Part model, mm, in its own coordinate system. A direction names the side the tool comes from. Round coordinates to 2 decimals unless told otherwise and drop trailing zeros. Loops run counter-clockwise (first coordinate to the right, second up) from the corner with the lowest first, then second, coordinate; pieces in that order, holes last.
1) Mould opens along Z. For faces 1 (the flat face through (-1.052, 23.271, 3.355)), 2 (the cylindrical face through (0.69, 9.39, 3.1)), 3 (the flat face through (-3.43, 23.27, 0.77)), 4 (the flat face through (0, 0, 0)) say: +Z half, -Z half, draft (parallel to the pull), parting line (faces both ways), or undercut.
2) 3-axis set-ups, long thin cutter, end or side, ignore diameter. For faces 5 (the flat face through (-2, 19.05, -3)), 6 (the flat face through (3, 25.4, 3)), 7 (the flat face through (1.052, 23.271, -3.355)): which of +Z, -Z, +X, -X, +Y, -Y reach the whole face in a straight line?
3) Drop flat-ended pins along their axis: P1, Ø4, axis at x = -2, z = -2, coming from the -Y side; P2, Ø4, axis at x = 0.5, y = 14.5, coming from the -Z side (3 decimals); P3, Ø4, axis at x = -0.5, y = 3, coming from the +Z side (3 decimals). Give the stop position or say it passes through.
4) Band-saw the part on A-A, the plane y = 18.5. Write the cut outline in (x, z) (3 decimals), then the cut area to 3 significant figures.
5) Band-saw the part on C-C, the plane z = 0. Write the cut outline in (x, y) (3 decimals).
6) Band-saw the part on D-D, the plane x = -3.5. Write the cut outline in (y, z), then the cut area to 3 significant figures.
7) Band-saw the part on B-B, the plane x = 0. Write the cut outline in (y, z) (3 decimals), then the cut area to 3 significant figures.
8) Probe line 1 (Y direction, x = -0.5, z = -2); line 2 (Y direction, x = -4, z = 0.5); line 3 (Z direction, x = -1, y = 14.25). List the from-to ranges inside material, lowest first.
Autodesk Inventor part; units mm, degrees
ref_plane "YZ Plane" through (0, 0, 0) normal (1, 0, 0) x (0, 1, 0)
ref_plane "XZ Plane" through (0, 0, 0) normal (0, 1, 0) x (-1, 0, 0)
ref_plane "XY Plane" through (0, 0, 0) normal (0, 0, 1) x (1, 0, 0)
sketch "Sketch1" plane through (0, 0, 0) normal (0, 1, 0) x (-1, 0, 0)
  circle A0 centre (0, 0) radius 3.175
  dimension "d2" = 6.35
extrude "Extrusion1" add sketch "Sketch1" along normal blind 19.05
thread "Thread1"
sketch "Sketch2" plane through (0, 19.05, 0) normal (0, 1, 0) x (1, 0, 0)
  circle A0 centre (0, 0) radius 6.35
  dimension "d7" = 12.7
extrude "Extrusion2" add sketch "Sketch2" along normal blind 6.35
sketch "Sketch3" plane through (0, 25.4, 0) normal (0, 1, 0) x (1, 0, 0)
  line L0 (3.0114, 2.7237) -> (3.8645, -1.2461)
  line L1 (3.8645, -1.2461) -> (0.8531, -3.9698)
  line L2 (0.8531, -3.9698) -> (-3.0114, -2.7237)
  line L3 (-3.0114, -2.7237) -> (-3.8645, 1.2461)
  line L4 (-3.8645, 1.2461) -> (-0.8531, 3.9698)
  line L5 (-0.8531, 3.9698) -> (3.0114, 2.7237)
  point P0 (0, 0)
  point P1 (0, 0)
extrude "Extrusion3" cut sketch "Sketch3" against normal blind 4.318
properties part number "qtr20_75"
Reported:
1. face 1: undercut
1. face 2: parting line
1. face 3: undercut
1. face 4: draft
2. face 5: -Y
2. face 6: +Z, -Z, +X, -X, +Y
2. face 7: +Y
3. P1: stops at y = 0
3. P2: stops at z = -3.175
3. P3: stops at z = 3.175
4. outline: circle Ø6.35 at (0, 0)
4. area: 31.7 mm2
5. outline: (-6.35, 19.05) - (-3.175, 19.05) - (-3.175, 0) - (3.175, 0) - (3.175, 19.05) - (6.35, 19.05) - (6.35, 25.4) - (3.597, 25.4) - (3.597, 21.082) - (-3.597, 21.082) - (-3.597, 25.4) - (-6.35, 25.4) - close
6. outline: (19.05, -5.3) - (25.4, -5.3) - (25.4, -1.58) - (21.08, -1.58) - (21.08, 0.45) - (25.4, 0.45) - (25.4, 5.3) - (19.05, 5.3) - close
6. area: 58.5 mm2
7. outline: (0, -3.175) - (19.05, -3.175) - (19.05, -6.35) - (25.4, -6.35) - (25.4, -3.695) - (21.082, -3.695) - (21.082, 3.695) - (25.4, 3.695) - (25.4, 6.35) - (19.05, 6.35) - (19.05, 3.175) - (0, 3.175) - close
7. area: 170 mm2
8. line 1: y = 0 to 21.08
8. line 2: y = 19.05 to 25.4
8. line 3: z = -3.01 to 3.01
